from build123d import *

# Parameters (mm, degrees)
BOSS_EXTRUDE1_DEPTH = 1.5875
BOSS_EXTRUDE2_DEPTH = 1.5875


with BuildPart() as part:
    # Sketch1 → Boss-Extrude1 (new body)
    with BuildSketch(Plane.XY):
        Polygon((-20, 20), (-20, 80), (20, 80), (20, 20), (80, 20), (80, -20), (20, -20), (20, -120), (-20, -120), (-20, -20), (-80, -20), (-80, 20), align=None)
    extrude(amount=BOSS_EXTRUDE1_DEPTH)

    # Sketch13 → Boss-Extrude2 (add)
    with BuildSketch(Plane.XY):
        Polygon((-80, 7.5), (-80, -7.5), (-81.4, -7.5), (-81.4, -10), (-87.5, -5), (-87.5, 5), (-81.4, 10), (-81.4, 7.5), align=None)
    extrude(amount=BOSS_EXTRUDE2_DEPTH)


solid = part.part
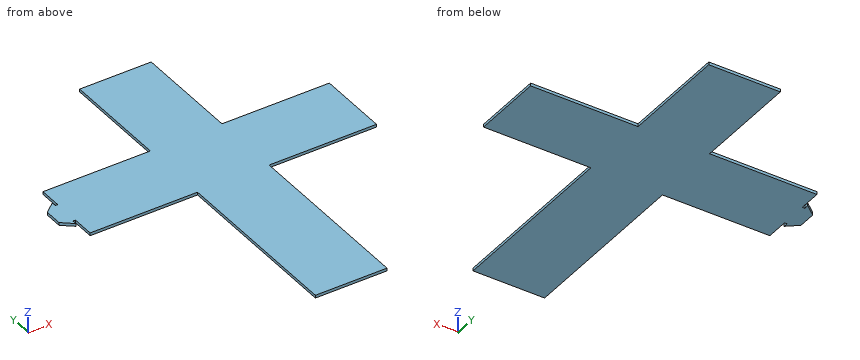
Can you work these out from the model? Positions are in its coordinate system, mm. Coordinates: 2 decimals unless noted, no trailing zeros. Write each loop counter-clockwise with the first axis right and the second up, starting at its lowest first coordinate (ties: lowest second). Pieces come first, ordered by that corner, then holes. Notation, with made-up numbers: (61, -25.75) -> (103, -25.75) arc R7 cw to (103, -21.75) -> close; hole circle Ø1 at (44, -19.75). An arc over 180 degrees is marked (long way). Write each question's results on one line, items separated by ' | '. Start each with the question number.
Q1. Imagine slicing it at C-C (y = -16.5). Write out the boundary of the cut face in (x, z), then the cut area to 3 significant figures.
Q2. Imagine slicing it at A-A (z = 0.95). Write out the boundary of the cut face in (x, y), then the cut area to 3 significant figures.
Q3. Imagine slicing it at B-B (x = 55). Write out the boundary of the cut face in (y, z), then the cut area to 3 significant figures.
Q4. I'm going to push flat-ended pins straight in: pin 1 (0.8 mm diameter, centred on y = 13, z = 0.5, fed in from -X); pin 2 (0.5 mm diameter, centred on x = -54.5, z = 1, fed in from +Y); pin 3 (0.5 mm diameter, centred on y = -46.5, z = 0.5, fed in from +X). Where does each tip first touch, or does it pass through?
Q5. If I drill on probe 1 along Y at (x, z) = (21.5, 0.7); probe 2 along X at (y, z) = (19.5, 0.4), over which ranges is the centre line in solid material (lowest first)?
Taken from the geometry:
1) outline: (-80, 0) -> (80, 0) -> (80, 1.59) -> (-80, 1.59) -> close | area: 254 mm^2
2) outline: (-87.5, -5) -> (-81.4, -10) -> (-81.4, -7.5) -> (-80, -7.5) -> (-80, -20) -> (-20, -20) -> (-20, -120) -> (20, -120) -> (20, -20) -> (80, -20) -> (80, 20) -> (20, 20) -> (20, 80) -> (-20, 80) -> (-20, 20) -> (-80, 20) -> (-80, 7.5) -> (-81.4, 7.5) -> (-81.4, 10) -> (-87.5, 5) -> close | area: 12,900 mm^2
3) outline: (-20, 0) -> (20, 0) -> (20, 1.59) -> (-20, 1.59) -> close | area: 63.5 mm^2
4) pin 1: stops at x = -80 | pin 2: stops at y = 20 | pin 3: stops at x = 20
5) probe 1: y = -20 to 20 | probe 2: x = -80 to 80
